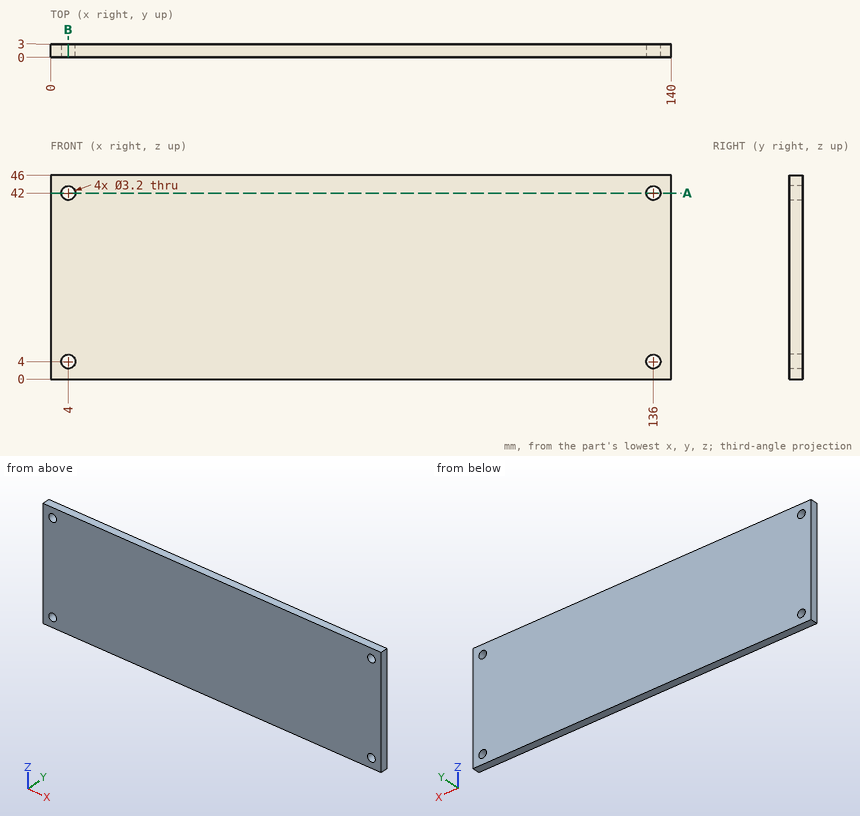
Part print with two shaded views. Sizes in mm from the minimum x, y, z corner. Coordinates: 2 decimals unless noted, no trailing zeros. Loops run counter-clockwise (first coordinate to the right, second up) from the corner with the lowest first, then second, coordinate; pieces in that order, holes last. Notation, with made-up numbers: (-14, -2.5) -> (16, -2.5) arc R10 cw to (16, 12.5) -> close; hole circle Ø9 at (59, 8.25). An arc over 180 degrees is marked (long way). Answer as a JSON object with one key per item and string values.
Q1. Cut at A-A (z = 42). List the corners of the cut face in (x, y), and give its area (3 significant figures).
Report:
{"outline": "(0, 0) -> (2.4, 0) -> (2.4, 3) -> (0, 3) -> close; (5.6, 0) -> (134.4, 0) -> (134.4, 3) -> (5.6, 3) -> close; (137.6, 0) -> (140, 0) -> (140, 3) -> (137.6, 3) -> close", "area": "401 mm2"}
Q2. Cut at B-B (x = 4). List the corners of the cut face in (y, z), and give its area (3 significant figures).
Report:
{"outline": "(0, 0) -> (3, 0) -> (3, 2.4) -> (0, 2.4) -> close; (0, 5.6) -> (3, 5.6) -> (3, 40.4) -> (0, 40.4) -> close; (0, 43.6) -> (3, 43.6) -> (3, 46) -> (0, 46) -> close", "area": "119 mm2"}
Q3. Flat gauge pin, fed straight in: P1, Ø3, axis at x = 136, z = 42, coming from the -Y side. Where does the tip first touch, or does it go through?
Report:
{"P1": "passes through"}
Q4. Probe probe 1 along Z at (x, y) = (4, 1.85); probe 2 along X at (y, z) = (2, 42); probe 3 along X at (y, z) = (0.3, 43). List the from-to ranges inside material, lowest first.
Report:
{"probe 1": "z = 0 to 2.4, 5.6 to 40.4, 43.6 to 46", "probe 2": "x = 0 to 2.4, 5.6 to 134.4, 137.6 to 140", "probe 3": "x = 0 to 2.75, 5.25 to 134.75, 137.25 to 140"}
